Verification items for the finished model (mm, model axes). Give positions to 0.01 mm unless a question says otherwise; leave off trailing zeros. Loops run counter-clockwise (first coordinate to the right, second up) from the corner with the lowest first, then second, coordinate; pieces in that order, holes last. Notation, with made-up numbers: (49, 42) -> (92, 42) arc R27 cw to (92, 68) -> close; hole circle Ø10 at (77.5, 67). An arc over 180 degrees is marked (long way). Answer in a Markdown table with one row per item. Add a question column.
Q1. Material ranges on probe 1 along Y at (x, z) = (6.6, -0.2); probe 2 along Z at (x, y) = (2.25, 82); probe 3 along X at (y, z) = (9.5, -4.25), recorded low to high.
Q2. Section check A-A on y = 71. Enter the section's corners in (x, z).
Q3. Gauge pin test, flat ends, axial feed: P1, Ø5, axis at x = -5.5, z = -2, coming from the -Y side; P2, Ø3, axis at x = -3.5, z = 1.5, coming from the +Y side. Record the tip position at first contact, or that the pin passes through.
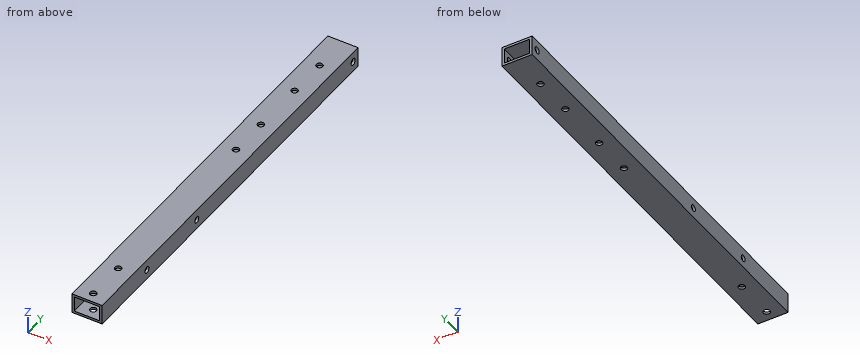
```python
from build123d import *

# Parameters (mm, degrees)
SKETCH_1_W          = 15
SKETCH_1_H          = 10
SKETCH_1_W_2        = 12.6
SKETCH_1_H_2        = 7.6
EXTRUDE_1_DEPTH     = 110
SKETCH_2_R          = 1.6
CUT_EXTRUDE_1_DEPTH = 100
SKETCH_3_R          = 1.6
CUT_EXTRUDE_2_DEPTH = 15
SKETCH_5_W          = 15
SKETCH_5_H          = 10
CUT_EXTRUDE_4_DEPTH = 14.5
SKETCH_6_R          = 1.6
CUT_EXTRUDE_5_DEPTH = 15
CUT_EXTRUDE_6_DEPTH = 15
SKETCH_8_R          = 1.6
CUT_EXTRUDE_7_DEPTH = 10


with BuildPart() as part:
    # ｽｹｯﾁ1 → ﾎﾞｽ - 押し出し1 (new, symmetric)
    with BuildSketch(Plane(origin=(0, 0, 0), x_dir=(1, 0, 0), z_dir=(0, 1, 0))):
        Rectangle(SKETCH_1_W, SKETCH_1_H)
        Rectangle(SKETCH_1_W_2, SKETCH_1_H_2, mode=Mode.SUBTRACT)
    extrude(amount=EXTRUDE_1_DEPTH, both=True)

    # ｽｹｯﾁ2 → ｶｯﾄ - 押し出し1 (cut)
    with BuildSketch(Plane(origin=(0, 0, -5), x_dir=(-1, 0, 0), z_dir=(0, 0, -1))):
        with Locations((0, -85)):
            Circle(SKETCH_2_R)
        with Locations((0, -105)):
            Circle(SKETCH_2_R)
    extrude(amount=-CUT_EXTRUDE_1_DEPTH, mode=Mode.SUBTRACT)

    # ｽｹｯﾁ3 → ｶｯﾄ - 押し出し2 (cut)
    with BuildSketch(Plane.ZY.offset(7.5)):
        with Locations((-0.2, -74)):
            Circle(SKETCH_3_R)
        with Locations((-0.2, -34)):
            Circle(SKETCH_3_R)
    extrude(amount=-CUT_EXTRUDE_2_DEPTH, mode=Mode.SUBTRACT)

    # ｽｹｯﾁ5 → ｶｯﾄ - 押し出し4 (cut)
    with BuildSketch(Plane(origin=(0, 110, 0), x_dir=(1, 0, 0), z_dir=(0, 1, 0))):
        Rectangle(SKETCH_5_W, SKETCH_5_H)
    extrude(amount=-CUT_EXTRUDE_4_DEPTH, mode=Mode.SUBTRACT)

    # ｽｹｯﾁ6 → ｶｯﾄ - 押し出し5 (cut)
    with BuildSketch(Plane(origin=(0, 0, -5), x_dir=(-1, 0, 0), z_dir=(0, 0, -1))):
        with Locations((0, 56.66)):
            Circle(SKETCH_6_R)
        with Locations((0, 76.66)):
            Circle(SKETCH_6_R)
    extrude(amount=-CUT_EXTRUDE_5_DEPTH, mode=Mode.SUBTRACT)

    # ｽｹｯﾁ7 → ｶｯﾄ - 押し出し6 (cut)
    with BuildSketch(Plane.ZY.offset(7.5)):
        with BuildLine():
            ThreePointArc((0, 93.15), (-1.65, 91.5), (0, 89.85))
            ThreePointArc((0, 89.85), (1.65, 91.5), (0, 93.15))
        make_face()
    extrude(amount=-CUT_EXTRUDE_6_DEPTH, mode=Mode.SUBTRACT)

    # ｽｹｯﾁ8 → ｶｯﾄ - 押し出し7 (cut)
    with BuildSketch(Plane(origin=(0, 0, -5), x_dir=(-1, 0, 0), z_dir=(0, 0, -1))):
        with Locations((0, 9.6)):
            Circle(SKETCH_8_R)
        with Locations((0, 29.6)):
            Circle(SKETCH_8_R)
    extrude(amount=-CUT_EXTRUDE_7_DEPTH, mode=Mode.SUBTRACT)


solid = part.part
```
Taken from the geometry:
| question | item | result |
|---|---|---|
| 1 | probe 1 | y = -110 to -75.6, -72.4 to -35.6, -32.4 to 89.86, 93.14 to 95.5 |
| 1 | probe 2 | z = -5 to -3.8, 3.8 to 5 |
| 1 | probe 3 | x = -7.5 to -1.6, 1.6 to 7.5 |
| 2 | outline | (-7.5, -5) -> (7.5, -5) -> (7.5, 5) -> (-7.5, 5) -> close; hole (-6.3, -3.8) -> (6.3, -3.8) -> (6.3, 3.8) -> (-6.3, 3.8) -> close |
| 3 | P1 | stops at y = -110 |
| 3 | P2 | passes through |
